from build123d import *

# Parameters (mm, degrees)
F1_DEPTH = 63.5
F0_W     = 25.4
F0_H     = 19.05
F2_DEPTH = 25.4
F3_DEPTH = 7.9375
F5_R     = 6.35


# Not quite as in the source:
# - a feature names something its author has since deleted; it is built from what else it names


with BuildPart() as f1:
    # F0 (on Front) → F1 (new body, symmetric)
    with BuildSketch(Plane.XZ):
        Polygon((-41.275, 9.525), (-41.275, -9.525), (41.275, -9.525), (41.275, 9.525), (22.225, 9.525), align=None)
    extrude(amount=F1_DEPTH, both=True)

    # F0 (on Front) → F2 (join, symmetric)
    with BuildSketch(Plane.XZ):
        with BuildLine():
            Line((22.225, 9.525), (41.275, 9.525))
            Line((41.275, 9.525), (41.275, 27.0002))
            ThreePointArc((41.275, 27.0002), (45.9246798487, 38.2255201513), (57.15, 42.8752))
            Line((57.15, 42.8752), (60.325, 42.8752))
            Line((60.325, 42.8752), (60.325, 61.9252))
            Line((60.325, 61.9252), (57.15, 61.9252))
            ThreePointArc((57.15, 61.9252), (32.4542956671, 51.6959043329), (22.225, 27.0002))
            Line((22.225, 27.0002), (22.225, 9.525))
        make_face()
        with Locations((73.025, 52.4002)):
            Rectangle(F0_W, F0_H)
    extrude(amount=F2_DEPTH, both=True)

    # F0 (on Front) → F3 (join, symmetric)
    with BuildSketch(Plane.XZ):
        with BuildLine():
            add(Edge.make_bspline(
                [(-41.275, 9.525), (-41.275, 40.5423477454), (8.4285710651, 61.9252), (57.15, 61.9252)],
                knots=[0, 0, 0, 0, 111.5045361635, 111.5045361635, 111.5045361635, 111.5045361635], degree=3))
            Line((-41.275, 9.525), (22.225, 9.525))
            Line((22.225, 9.525), (22.225, 27.0002))
            ThreePointArc((22.225, 27.0002), (32.4542956671, 51.6959043329), (57.15, 61.9252))
        make_face()
    extrude(amount=F3_DEPTH, both=True)

    # F0 (on Front) → F4 (revolve)
    with BuildSketch(Plane.XZ):
        Polygon((85.725, 66.675), (85.725, 61.9252), (85.725, 42.8752), (85.725, 38.1), (111.125, 38.1), (111.125, 66.675), align=None)
    revolve(axis=Axis((85.725, 0, 52.3875), (0, 0, 1)))

    # F5
    f5_edges = [f1.edges().sort_by_distance(p)[0] for p in [
        (41.275, -63.5, 0),
        (-41.275, -63.5, 0),
        (41.275, 63.5, 0),
        (-41.275, 63.5, 0),
    ]]
    fillet(f5_edges, radius=F5_R)


solid = f1.part
Read the model definition and answer for the solid it produces. Units are mm, in the model's axes. A direction names the side the tool comes from. Give positions to 0.01 mm unless a question says otherwise; leave off trailing zeros. Write each loop counter-clockwise with the first axis right and the second up, starting at its lowest first coordinate (ties: lowest second). Pieces come first, ordered by that corner, then holes. Notation, with made-up numbers: (69, -5) - (112, -5) arc R13 ccw to (112, 12) - close; hole circle Ø8 at (-17, -1). An arc over 180 degrees is marked (long way). Answer in a Markdown table with one row per item. Add a question column.
Item 1: Section A-A, the plane x = 67 is taken. Write down the section's boundary in (y, z) (3 decimals), and give its area (3 significant figures).
Item 2: Section B-B, the plane y = 21.5 is taken. Write down the section's boundary in (x, z) (3 decimals).
Item 3: A tool of negligible diameter and unlimited length cuts with its end or side. For faces 1 (the face through (46, 25.4, 42)), 2 (the face through (22.225, -17, 18)), 3 (the face through (32.73, 16.55, 51.97)), 4 (the face through (86, 0, 38.1)), 5 (the face through (60, 2, 42.875)), from which of +Z, -Z, +X, -X, +Y, -Y can it reach the whole face along a straight path? Write none if from no direction.
Item 4: Flat-ended cylindrical pins translate along their axes: P1, Ø5, axis at y = -17, z = 15.5, coming from the -X side (3 decimals); P2, Ø18.5, axis at y = -24, z = 11.5, coming from the +X side (3 decimals); P3, Ø14.5, axis at x = 73, y = -3, coming from the -Z side. Find the tip coordinate at first contact, or state that the pin passes through.
Item 5: Find the intervals of material crossed by L1, parallel to X at y = -19.5, z = -1 (3 decimals); L2, parallel to Y at x = 84, z = 58; L3, parallel to Y at x = 22, z = 35, in increasing order.
Item 6: Section C-C, the plane y = -18 is taken. Write down the section's boundary in (x, z) (3 decimals), and give its area (3 significant figures).
Recorded:
| question | item | result |
|---|---|---|
| 1 | outline | (-25.4, 42.875) - (-17.162, 42.875) - (-17.162, 38.1) - (17.162, 38.1) - (17.162, 42.875) - (25.4, 42.875) - (25.4, 61.925) - (17.162, 61.925) - (17.162, 66.675) - (-17.162, 66.675) - (-17.162, 61.925) - (-25.4, 61.925) - close |
| 1 | area | 1,290 mm2 |
| 2 | outline | (-41.275, -9.525) - (41.275, -9.525) - (41.275, 27) arc R15.875 cw to (57.15, 42.875) - (72.201, 42.875) - (72.201, 38.1) - (99.249, 38.1) - (99.249, 66.675) - (72.201, 66.675) - (72.201, 61.925) - (57.15, 61.925) arc R34.925 ccw to (22.225, 27) - (22.225, 9.525) - (-41.275, 9.525) - close |
| 3 | face 1 | +Z, +X, -X, +Y |
| 3 | face 2 | +Z, -X, -Y |
| 3 | face 3 | +Z, -X, +Y |
| 3 | face 4 | -Z, +X, +Y, -Y |
| 3 | face 5 | -Z |
| 4 | P1 | stops at x = 22.225 |
| 4 | P2 | stops at x = 41.275 |
| 4 | P3 | stops at z = 38.1 |
| 5 | L1 | x = -41.275 to 41.275 |
| 5 | L2 | y = -25.4 to 25.4 |
| 5 | L3 | y = -7.94 to 7.94 |
| 6 | outline | (-41.275, -9.525) - (41.275, -9.525) - (41.275, 27) arc R15.875 cw to (57.15, 42.875) - (67.804, 42.875) - (67.804, 38.1) - (103.646, 38.1) - (103.646, 66.675) - (67.804, 66.675) - (67.804, 61.925) - (57.15, 61.925) arc R34.925 ccw to (22.225, 27) - (22.225, 9.525) - (-41.275, 9.525) - close |
| 6 | area | 3,890 mm2 |
